```python
from build123d import *

# Parameters (mm, degrees)
CROQUIS1_R              = 1.55
SALIENTE_EXTRUIR2_DEPTH = 8
REDONDEO1_R             = 8
REDONDEO2_R             = 5
CROQUIS2_R              = 2.8
CORTAR_EXTRUIR1_DEPTH   = 1
CROQUIS3_W              = 8
CROQUIS3_H              = 31
SALIENTE_EXTRUIR3_DEPTH = 12
CROQUIS4_R              = 1.55
CORTAR_EXTRUIR2_DEPTH   = 8
CORTAR_EXTRUIR3_DEPTH   = 2.5
REDONDEO3_R             = 1.5
REDONDEO4_R             = 1.5
CHAFL_N1_SIZE           = 3.8


with BuildPart() as part:
    # Croquis1 → Saliente-Extruir2 (new body)
    with BuildSketch(Plane(origin=(0, 0, 0), x_dir=(1, 0, 0), z_dir=(0, 1, 0))):
        with BuildLine():
            Line((0, 0), (42, 0))
            Line((42, 0), (42, 36.5))
            ThreePointArc((42, 36.5), (37.234408514, 41.950747117), (31.196129406, 37.95566367))
            ThreePointArc((31.196129406, 37.95566367), (26.790448284, 33.865529217), (21, 32.25))
            ThreePointArc((21, 32.25), (32.25, 21), (21, 9.75))
            ThreePointArc((21, 9.75), (10.169247694, 11.081546284), (0, 15.039400798))
            Line((0, 15.039400798), (0, 0))
        make_face()
        with Locations((36.5, 36.5)):
            Circle(CROQUIS1_R, mode=Mode.SUBTRACT)
        with Locations((5.5, 5.5)):
            Circle(CROQUIS1_R, mode=Mode.SUBTRACT)
    extrude(amount=SALIENTE_EXTRUIR2_DEPTH)

    # Redondeo1
    redondeo1_edges = [part.edges().sort_by_distance(p)[0] for p in [
        (21, 4, -32.25),
    ]]
    fillet(redondeo1_edges, radius=REDONDEO1_R)

    # Redondeo2
    redondeo2_edges = [part.edges().sort_by_distance(p)[0] for p in [
        (0, 4, -15.039400798),
    ]]
    fillet(redondeo2_edges, radius=REDONDEO2_R)

    # Croquis2 → Cortar-Extruir1 (cut)
    with BuildSketch(Plane(origin=(0, 8, 0), x_dir=(1, 0, 0), z_dir=(0, 1, 0))):
        with Locations((36.5, 36.5)):
            Circle(CROQUIS2_R)
        with Locations((5.5, 5.5)):
            Circle(CROQUIS2_R)
    extrude(amount=-CORTAR_EXTRUIR1_DEPTH, mode=Mode.SUBTRACT)

    # Croquis3 → Saliente-Extruir3 (add)
    with BuildSketch(Plane(origin=(0, 8, 0), x_dir=(1, 0, 0), z_dir=(0, 1, 0))):
        with Locations((38, 15.5)):
            Rectangle(CROQUIS3_W, CROQUIS3_H)
    extrude(amount=SALIENTE_EXTRUIR3_DEPTH)

    # Croquis4 → Cortar-Extruir2 (cut)
    with BuildSketch(Plane.ZY.offset(-34)):
        with Locations((-25, 14)):
            Circle(CROQUIS4_R)
        with Locations((-5, 14)):
            Circle(CROQUIS4_R)
    extrude(amount=-CORTAR_EXTRUIR2_DEPTH, mode=Mode.SUBTRACT)

    # Croquis5 → Cortar-Extruir3 (cut)
    with BuildSketch(Plane.ZY.offset(-34)):
        Polygon((-25, 17.348631561), (-27.9, 15.674315781), (-27.9, 12.325684219), (-25, 10.651368439), (-22.1, 12.325684219), (-22.1, 15.674315781), align=None)
        Polygon((-5, 17.348631561), (-7.9, 15.674315781), (-7.9, 12.325684219), (-5, 10.651368439), (-2.1, 12.325684219), (-2.1, 15.674315781), align=None)
    extrude(amount=-CORTAR_EXTRUIR3_DEPTH, mode=Mode.SUBTRACT)

    # Redondeo3
    redondeo3_edges = [part.edges().sort_by_distance(p)[0] for p in [
        (34, 8, -15.5),
    ]]
    fillet(redondeo3_edges, radius=REDONDEO3_R)

    # Redondeo4
    redondeo4_edges = [part.edges().sort_by_distance(p)[0] for p in [
        (38, 20, -31),
        (38, 20, 0),
    ]]
    fillet(redondeo4_edges, radius=REDONDEO4_R)

    # Chaflán1
    chafl_n1_edges = [part.edges().sort_by_distance(p)[0] for p in [
        (0, 4, 0),
    ]]
    chamfer(chafl_n1_edges, length=CHAFL_N1_SIZE)


solid = part.part
```
Verification items for the finished model (mm, model axes). A direction names the side the tool comes from. Round coordinates to 2 decimals unless told otherwise and drop trailing zeros. Loops run counter-clockwise (first coordinate to the right, second up) from the corner with the lowest first, then second, coordinate; pieces in that order, holes last. Notation, with made-up numbers: (54.25, 88) -> (62.25, 88) arc R26 ccw to (62.25, 102) -> close; hole circle Ø8 at (56.25, 40). An arc over 180 degrees is marked (long way). Answer as a JSON object with one key per item and string values.
Q1. Section check C-C (y = 16.5). Record the boundary of the cut face in (x, z), then the cut area to 3 significant figures.
Data:
{"outline": "(34, -31) -> (42, -31) -> (42, 0) -> (34, 0) -> (34, -3.53) -> (36.5, -3.53) -> (36.5, -6.47) -> (34, -6.47) -> (34, -23.53) -> (36.5, -23.53) -> (36.5, -26.47) -> (34, -26.47) -> close", "area": "233 mm2"}
Q2. Access from +Z, -Z, +X, -X, +Y, -Y to the whole of each face (thin tool, end or side, straight path). Record for faces 5 (the flat face through (38, 7, -35)), 6 (the flat face through (35.232, 16.523, -26.43)), 7 (the cylindrical face through (13.814, 3.944, -10.326)), 8 (the flat face through (38, 13, -31)), 9 (the flat face through (1.9, 3.9, -1.9)).
Data:
{"face 5": "+Y", "face 6": "-X", "face 7": "-Z, +Y, -Y", "face 8": "-Z, +X, -X, +Y", "face 9": "+Z, -X, +Y, -Y"}
Q3. Section check B-B (z = -17). Record the boundary of the cut face in (x, y).
Data:
{"outline": "(31.51, 0) -> (42, 0) -> (42, 20) -> (34, 20) -> (34, 9.5) arc R1.5 cw to (32.5, 8) -> (31.51, 8) -> close"}
Q4. Scan lines: line 1 (Y direction, x = 38, z = -25); line 2 (X direction, y = 7.8, z = -5.5); line 3 (Y direction, x = 25.5, z = -1.5). Record each from-to range of solid material in increasing order. Write a range as from..to.
Data:
{"line 1": "y = 0..12.45, 15.55..20", "line 2": "x = 0..2.7, 8.3..42", "line 3": "y = 0..8"}
Q5. Section check A-A (x = 5.5). Record the boundary of the cut face in (y, z), then the cut area to 3 significant figures.
Data:
{"outline": "(0, -12.38) -> (8, -12.38) -> (8, -8.3) -> (7, -8.3) -> (7, -7.05) -> (0, -7.05) -> close; (0, -3.95) -> (7, -3.95) -> (7, -2.7) -> (8, -2.7) -> (8, 0) -> (0, 0) -> close", "area": "71.7 mm2"}
Q6. Section check D-D (x = 23.5). Record the boundary of the cut face in (y, z), then the cut area to 3 significant figures.
Data:
{"outline": "(0, -10.03) -> (8, -10.03) -> (8, 0) -> (0, 0) -> close", "area": "80.3 mm2"}
Q7. Draft check along Y on faces 1 (the flat face through (22, 8, -9)), 2 (the flat face through (42, 10, -18)), 3 (the flat face through (35, 14, -27.9)), 4 (the flat face through (30, 0, -12)). Enter one of: pulls with the +Y half, pulls with the -Y half, needs draft (parallel to the pull), parting line crosses it, or undercut.
Data:
{"face 1": "pulls with the +Y half", "face 2": "needs draft", "face 3": "undercut", "face 4": "pulls with the -Y half"}
Q8. Go/stop test with flat-tipped pins: P1, Ø2, axis at y = 14, z = -33, coming from the -X side; P2, Ø2, axis at x = 35.5, y = 13.5, coming from the -Z side; P3, Ø4.5, axis at x = 36.5, z = -36.5, coming from the -Y side; P4, Ø5, axis at x = 5.5, z = -5.5, coming from the +Y side. Record where each tip stops, or that it passes through.
Data:
{"P1": "passes through", "P2": "stops at z = -31", "P3": "stops at y = 0", "P4": "stops at y = 7"}
